```python
from build123d import *

# Parameters (mm, degrees)
BOSS_EXTRUDE1_DEPTH     = 30.48
SKETCH3_R               = 24.13
CUT_EXTRUDE4_DEPTH      = 90.914560616
SKETCH4_R               = 3.175
CUT_EXTRUDE5_DEPTH      = 63.754
CIRPATTERN3_COUNT       = 6
BOSS_EXTRUDE3_START     = -21.59
SKETCH8_R               = 2.54
BOSS_EXTRUDE3_DEPTH     = 21.59
CUT_EXTRUDE7_DEPTH      = 98.433832269
CUT_EXTRUDE7_DEPTH_BACK = 98.433832269
SKETCH9_W               = 7.62
SKETCH9_H               = 7.694027115
SKETCH10_W              = 0.762
SKETCH10_H              = 7.694027115
CUT_EXTRUDE8_DEPTH      = 21.59
FILLET1_R               = 2.54


with BuildPart() as part:
    # Sketch1 → Boss-Extrude1 (new body)
    with BuildSketch(Plane(origin=(0, 0, 0), x_dir=(1, 0, 0), z_dir=(0, 1, 0))):
        with BuildLine():
            Line((-78.958715675, 0), (-17.998715675, 0))
            ThreePointArc((-17.998715675, 0), (-48.478715675, 30.349942827), (-78.958715675, 0))
        make_face()
    extrude(amount=BOSS_EXTRUDE1_DEPTH)

    # Sketch3 → Cut-Extrude4 (cut, through all)
    with BuildSketch(Plane(origin=(0, 0, 0), x_dir=(1, 0, 0), z_dir=(0, 1, 0))):
        with Locations((-48.478715675, 0)):
            Circle(SKETCH3_R)
    extrude(amount=CUT_EXTRUDE4_DEPTH, mode=Mode.SUBTRACT)

    # Sketch4 → Cut-Extrude5 (cut)
    with BuildSketch(Plane.XY):
        with Locations((-48.824364134, 15.798935299)):
            Circle(SKETCH4_R)
    cut_extrude5 = extrude(amount=-CUT_EXTRUDE5_DEPTH, mode=Mode.SUBTRACT)

    # CirPattern3: Cut-Extrude5 ×6 about axis
    cirpattern3_axis = Axis((-48.478715675, 30.48, 0.130335837), (0, -1, 0))
    for i in range(1, CIRPATTERN3_COUNT):
        add(cut_extrude5.rotate(cirpattern3_axis, i * 360 / CIRPATTERN3_COUNT), mode=Mode.SUBTRACT)

    # Sketch8 → Boss-Extrude3 (add)
    with BuildSketch(Plane(origin=(0, 30.48, 0), x_dir=(1, 0, 0), z_dir=(0, 1, 0)).offset(BOSS_EXTRUDE3_START)):
        with BuildLine():
            ThreePointArc((-85.222855562, 3.454304155), (-85.663790647, -3.212512214), (-79.805409512, 0))
            Line((-79.805409512, 0), (-78.958715675, 0))
            ThreePointArc((-78.958715675, 0), (-78.797525927, 3.002894504), (-78.341212544, 5.975290109))
            Line((-78.341212544, 5.975290109), (-78.958715675, 5.975290109))
            Line((-78.958715675, 5.975290109), (-79.805409512, 5.975290109))
            Line((-79.805409512, 5.975290109), (-85.222855562, 3.454304155))
        make_face()
        with Locations(Location((-83.615409512, 0, 0), (0, 0, 270))):
            Circle(SKETCH8_R, mode=Mode.SUBTRACT)
    extrude(amount=BOSS_EXTRUDE3_DEPTH)

    # Sketch9 → Cut-Extrude7 (cut, two sides: drawn at the far end of the back side and taken through both)
    with BuildSketch(Plane.XY.offset(-CUT_EXTRUDE7_DEPTH_BACK)):
        with Locations((-83.615409512, 26.632986443)):
            Rectangle(SKETCH9_W, SKETCH9_H)
    extrude(amount=CUT_EXTRUDE7_DEPTH + CUT_EXTRUDE7_DEPTH_BACK, mode=Mode.SUBTRACT)

    # Sketch10 → Cut-Extrude8 (cut)
    with BuildSketch(Plane.XY):
        with Locations((-79.424409512, 26.632986443)):
            Rectangle(SKETCH10_W, SKETCH10_H)
    extrude(amount=-CUT_EXTRUDE8_DEPTH, mode=Mode.SUBTRACT)

    # Fillet1
    fillet1_edges = [part.edges().sort_by_distance(p)[0] for p in [
        (-48.478715675, 30.48, -24.13),
    ]]
    fillet(fillet1_edges, radius=FILLET1_R)


solid = part.part
```
Work out the finished part from the listing and answer in its coordinate system (mm). A direction names the side the tool comes from. Round coordinates to 2 decimals unless told otherwise and drop trailing zeros. Write each loop counter-clockwise with the first axis right and the second up, starting at its lowest first coordinate (ties: lowest second). Pieces come first, ordered by that corner, then holes.
1) Flat-ended cylindrical pins translate along their axes: P1, Ø1.8, axis at y = 28.5, z = -4, coming from the -X side; P2, Ø1.9, axis at x = -22, y = 14, coming from the +Z side; P3, Ø9, axis at x = -84, z = 0, coming from the +Y side; P4, Ø4.5, axis at x = -83.62, z = 0, coming from the -Y side. Find the tip coordinate at first contact, or state that the pin passes through.
2) A cutting plane is placed at B-B on y = 25. Determine the outline of the cut face in (x, z), and give its area (3 significant figures).
3) A cutting plane is placed at C-C on y = 11. Determine the outline of the cut face in (x, z).
4) A cutting plane is placed at A-A on z = 1. Determine the outline of the cut face in (x, y), and give its area (3 significant figures).
5) Determine the mould class of faces 1 (the face through (-85.76, 15.74, 3.15)), 2 (the face through (-72.51, 12.7, -12.55)), 3 (the face through (-21, 15, 0)) for opening direction Z: pulls with the +Z half, pulls with the -Z half, needs draft (parallel to the pull), parting line crosses it, or undercut.
6) Consider probe 1 along Z at (x, y) = (-49, 28); probe 2 along X at (y, z) = (15, -8.5); probe 3 along X at (y, z) = (6.5, -1). Determine where each line is inside the solid, lowest interval first.
7) Which of the six approach directions +Z, -Z, +X, -X, +Y, -Y give full straight-line access (tool end or side, diameter ignored) to faces 4 (the face through (-76, 15, 0)), 5 (the face through (-79, 17, -5.975)), 6 (the face through (-81, 22.786, -2))?
Entries:
1. P1: stops at x = -79.04
1. P2: stops at z = 0
1. P3: stops at y = 22.79
1. P4: passes through
2. outline: (-79.04, -5.98) - (-78.34, -5.98) arc R30.48 ccw to (-18, 0) - (-24.35, 0) arc R24.13 cw to (-72.61, 0) - (-79.04, 0) - close
2. area: 539 mm2
3. outline: (-85.22, -3.45) - (-79.81, -5.98) - (-78.34, -5.98) arc R30.48 ccw to (-18, 0) - (-24.35, 0) arc R24.13 cw to (-72.61, 0) - (-79.81, 0) arc R3.81 ccw (long way) to start; hole circle Ø5.08 at (-83.62, 0)
4. outline: (-87.29, 8.89) - (-85.95, 8.89) - (-85.95, 22.79) - (-87.29, 22.79) - close; (-81.28, 8.89) - (-79.94, 8.89) - (-79.94, 22.79) - (-81.28, 22.79) - close
4. area: 37.3 mm2
5. face 1: parting line crosses it
5. face 2: undercut
5. face 3: pulls with the +Z half
6. probe 1: z = -30.35 to -24.13
6. probe 2: x = -77.71 to -71.06, -25.9 to -19.25
6. probe 3: x = -78.94 to -72.59, -24.37 to -18.02
7. face 4: +Z, +X, +Y, -Y
7. face 5: -Z, -X, +Y, -Y
7. face 6: +Z, -Z, -X, +Y
